Part print with two shaded views. Sizes in mm from the minimum x, y, z corner. Round coordinates to 2 decimals unless told otherwise and drop trailing zeros. Loops run counter-clockwise (first coordinate to the right, second up) from the corner with the lowest first, then second, coordinate; pieces in that order, holes last. Notation, with made-up numbers: (-14, 0.5) - (-2, 0.5) arc R30 cw to (-2, 39.5) - close; hole circle Ø5 at (-21, -15.75). An arc over 180 degrees is marked (long way). Put each result on its own line as item: value. Start each with the question number.
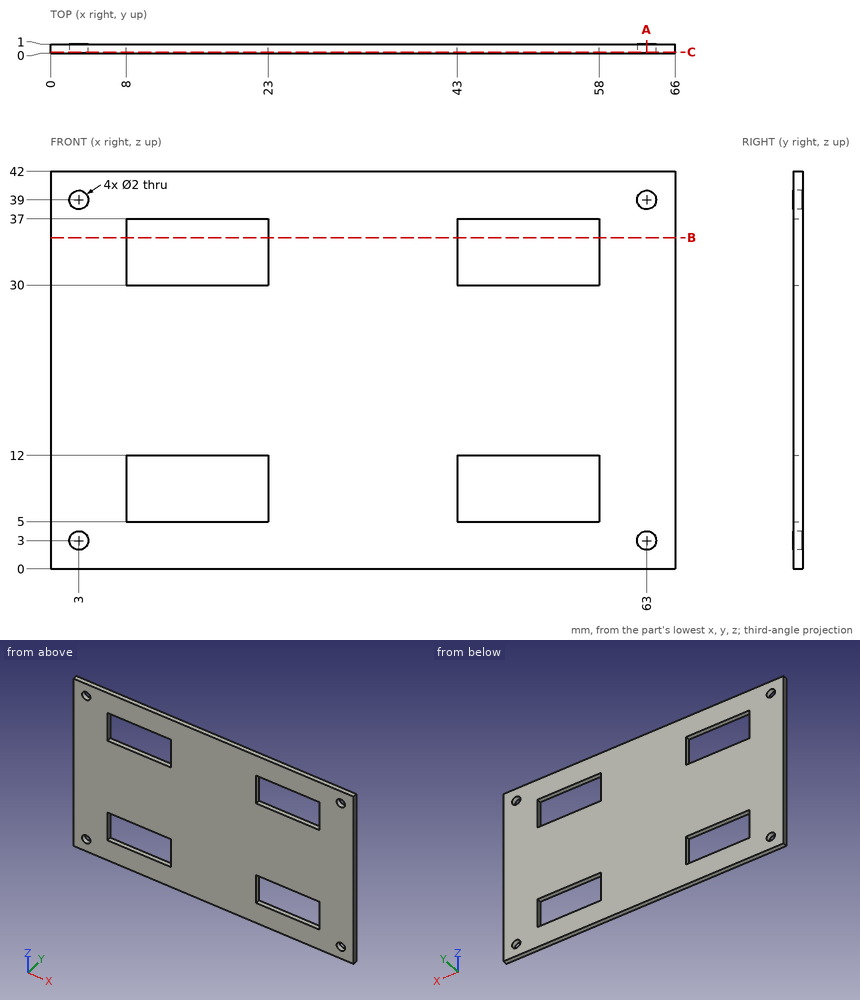
1) Drill centre lines: line 1 (Z direction, x = 63, y = 0.75); line 2 (X direction, y = 0.25, z = 32); line 3 (Z direction, x = 54.5, y = 0.5). Where is each one in solid material? Low to high. Write a range as [from, to].
2) Slice it at C-C, the plane y = 0.15. State how many separate pieces and enclosed holes the cut face has, and give its area (3 significant figures).
3) Slice it at A-A, the plane x = 63. Write the cut outline in (y, z).
4) Slice it at B-B, the plane z = 35. Write the cut outline in (x, y), and give its area (3 significant figures).
Taken from the geometry:
1. line 1: z = [0, 2], [4, 38], [40, 42]
1. line 2: x = [0, 8], [23, 43], [58, 66]
1. line 3: z = [0, 5], [12, 30], [37, 42]
2. separate pieces: 1
2. enclosed holes: 8
2. area: 2,340 mm2
3. outline: (0, 0) - (1, 0) - (1, 2) - (0, 2) - close; (0, 4) - (1, 4) - (1, 38) - (0, 38) - close; (0, 40) - (1, 40) - (1, 42) - (0, 42) - close
4. outline: (0, 0) - (8, 0) - (8, 1) - (0, 1) - close; (23, 0) - (43, 0) - (43, 1) - (23, 1) - close; (58, 0) - (66, 0) - (66, 1) - (58, 1) - close
4. area: 36.0 mm2
